Drawing for the job (mm, zero at the part's lowest x, y, z). Round coordinates to 2 decimals unless told otherwise and drop trailing zeros. Loops run counter-clockwise (first coordinate to the right, second up) from the corner with the lowest first, then second, coordinate; pieces in that order, holes last. Notation, with made-up numbers: M 67.5,42 L 78.5,42 A18 cw 78.5,67 Z; hole C -5,-12.75 d10. An arc over 180 degrees is marked long. Write each question's results on one line, items separated by ' | '.
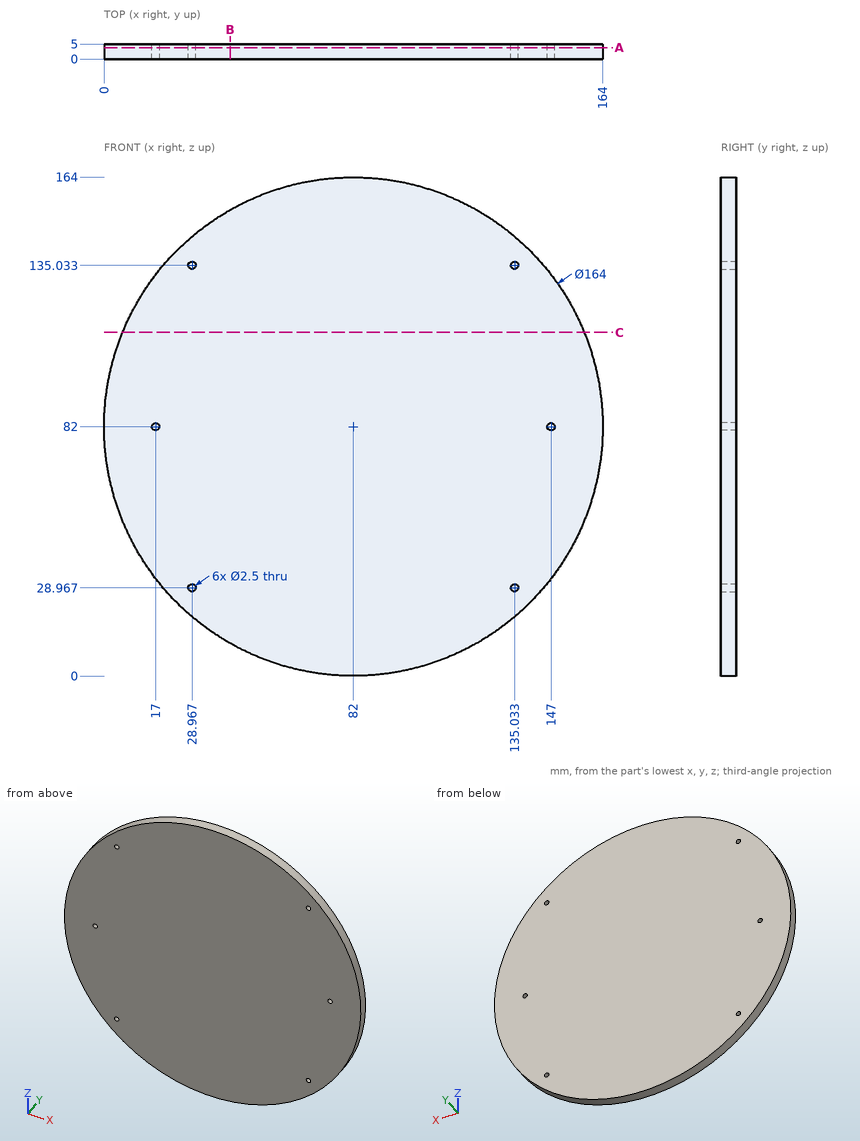
Item 1: Band-saw the part on A-A on y = 3.8. Give the cut face in (x, z), and give its area (3 significant figures).
Filled sheet:
outline: C 82,82 d164; hole C 17,82 d2.5; hole C 28.97,28.97 d2.5; hole C 28.97,135.03 d2.5; hole C 135.03,28.97 d2.5; hole C 135.03,135.03 d2.5; hole C 147,82 d2.5 | area: 21,100 mm^2
Item 2: Band-saw the part on C-C on z = 113. Give the cut face in (x, y).
Filled sheet:
outline: M 6.09,0 L 157.91,0 L 157.91,5 L 6.09,5 Z
Item 3: Band-saw the part on B-B on x = 41.5. Give the cut face in (y, z), and give its area (3 significant figures).
Filled sheet:
outline: M 0,10.7 L 5,10.7 L 5,153.3 L 0,153.3 Z | area: 713 mm^2
Item 4: Drop flat-ended pins along their axis: P1, Ø4, axis at x = 135.03, z = 135.03, coming from the +Y side; P2, Ø2, axis at x = 28.97, z = 135.03, coming from the +Y side; P3, Ø1.5, axis at y = 1.5, z = 73, coming from the +X side. Give the stop position or say it passes through.
Filled sheet:
P1: y = 5 | P2: through | P3: x = 163.58
Item 5: Wall check: L1, parallel to X at y = 3.6, z = 82; L2, parallel to X at y = 3.9, z = 81.5; L3, parallel to Z at x = 146.5, y = 3. Give the ranges that are in metal, low to high.
Filled sheet:
L1: 0 to 15.75, 18.25 to 145.75, 148.25 to 164 | L2: 0 to 15.85, 18.15 to 145.85, 148.15 to 164 | L3: 31.37 to 80.85, 83.15 to 132.63
